The drawing under review shows one solid part. Ordinate dimensions are in mm from its lowest x, y, z. Give positions to 0.01 mm unless a question says otherwise; leave off trailing zeros. Write each loop counter-clockwise with the first axis right and the second up, starting at its lowest first coordinate (ties: lowest second). Pieces come first, ordered by that corner, then holes. Notation, with made-up numbers: M 28,47 L 79,47 A27 ccw 79,83 Z; hole C -4,66 d1. An arc over 180 degrees is marked long. Write item = value, one per line. Start each with the question number.
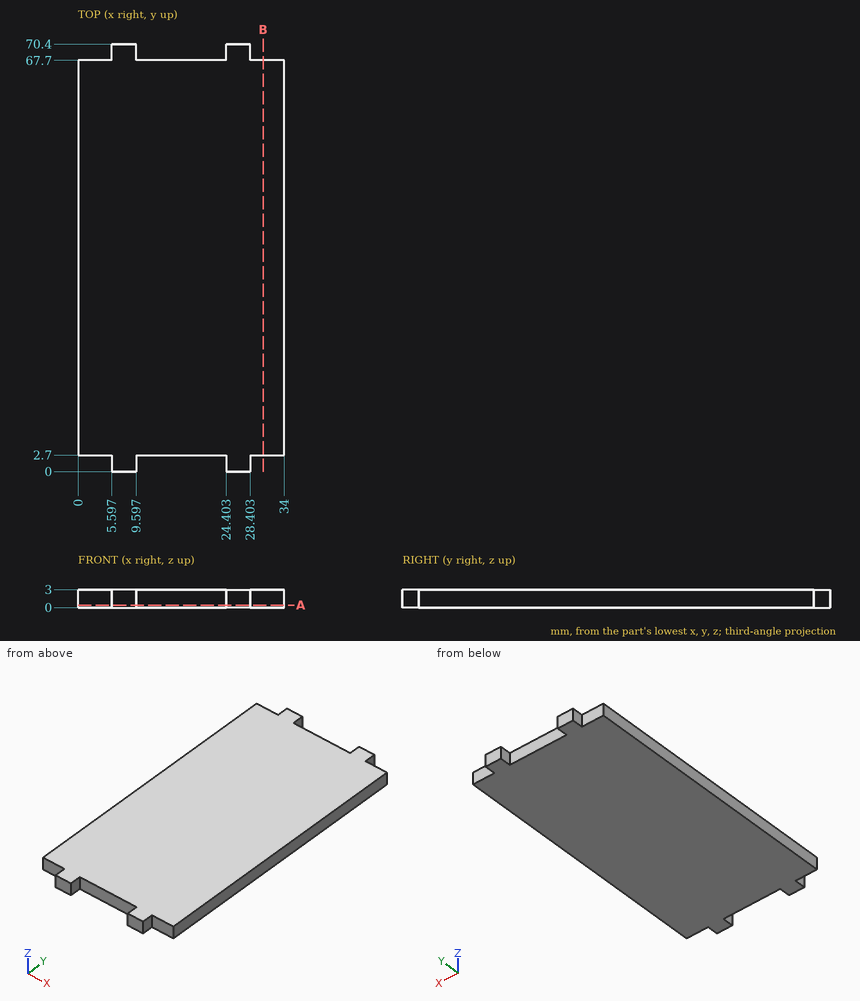
Item 1: We need section B-B, the plane x = 30.5. Write out the cut boundary in (y, z).
Item 2: To check wall thickness, follow probe 1 along Y at (x, z) = (11.5, 0.95). State the ranges of the line that lie inside material, in increasing order. Write a range as [from, to].
Item 3: We need section A-A, the plane z = 0.45. Write out the cut boundary in (x, y), and give its area (3 significant figures).
Item 4: Clearance check with flat-ended pins moving along their axes: P1, Ø0.8, axis at y = 68.5, z = 2, coming from the +X side; P2, Ø1.5, axis at x = 17, z = 1.5, coming from the +Y side; P3, Ø1.4, axis at y = 69.5, z = 2, coming from the -X side. State where each tip first meets the part, or that it passes through.
Worked out:
q1.outline = M 2.7,0 L 67.7,0 L 67.7,3 L 2.7,3 Z
q2.probe_1 = [2.7, 67.7]
q3.outline = M 0,2.7 L 5.6,2.7 L 5.6,0 L 9.6,0 L 9.6,2.7 L 24.4,2.7 L 24.4,0 L 28.4,0 L 28.4,2.7 L 34,2.7 L 34,67.7 L 28.4,67.7 L 28.4,70.4 L 24.4,70.4 L 24.4,67.7 L 9.6,67.7 L 9.6,70.4 L 5.6,70.4 L 5.6,67.7 L 0,67.7 Z
q3.area = 2,250 mm²
q4.P1 = 28.4
q4.P2 = 67.7
q4.P3 = 5.6
